Could you check a few things on this model? Use its own coordinates, in mm. A direction names the side the tool comes from. Coordinates: 2 decimals unless noted, no trailing zeros. Order: outer loops, then holes, each group sorted by start corner. A loop starts at its lowest first (then second) coordinate and runs counter-clockwise, first axis right, second up. Notation, with made-up numbers: (82.5, -23) - (99.5, -23) arc R29 cw to (99.5, 1) - close; hole circle Ø9 at (60.25, -35). An arc over 180 degrees is marked (long way). One line per item, written item: value. Start each with the question number.
from build123d import *

# Parameters (mm, degrees)
F1_DEPTH = 3
F2_D     = 3


# Not quite as in the source:
# - a feature names something its author has since deleted; it is built from what else it names


with BuildPart() as f1:
    # F0 (on Top) → F1 (new body)
    with BuildSketch(Plane.XY):
        Polygon((0, 31), (0, 0), (-35, 0), (-35, -15), (0, -15), (16, -15), (16, 31), align=None)
    extrude(amount=F1_DEPTH)

    # F2 (through all)
    with Locations(Plane(origin=(0, 0, 0), x_dir=(1, 0, 0), z_dir=(0, 0, -1))):
        with Locations((8, -8), (8, -22), (-10, 7.5), (-30, 7.5), (8, 6), (8, -26), (8, 10)):
            Hole(F2_D / 2)


solid = f1.part
Q1. I want a section at D-D on x = -21. Please give me the cut outline in (y, z), then the cut area to 3 significant figures.
Q2. I want a section at A-A on x = -30. Please give me the cut outline in (y, z).
Q3. If I drill on L1, parallel to Y at x = 8, z = 1.4; L2, parallel to Y at x = -30, z = 1.15; L3, parallel to X at y = -10, z = 0.7, over which ranges is the centre line in solid material (lowest first)?
Q4. I want a section at C-C on z = 2.1. Please give me the cut outline in (x, y).
Q5. Which directions (+Z, -Z, +X, -X, +Y, -Y) give clear straight access to the entire face, cutting with the end or side of a thin tool? Please do faces 5 (the flat face through (-17, 0, 1)), 6 (the cylindrical face through (8.195, 24.513, 1.521)).
Q6. We'd pull the mould along X, two halves only. Please class faces 1 (the flat face through (16, 8, 1)), 2 (the flat face through (0, 16, 1)), 3 (the flat face through (8, 31, 1)), 4 (the cylindrical face through (-28.5, -7.57, 1.52)): +X half, -X half, draft (parallel to the pull), parting line (faces both ways), or undercut.
Q7. I'm going to push flat-ended pins straight in: pin 1 (1.8 mm diameter, centred on x = 8, y = 8, fed in from -Z); pin 2 (0.9 mm diameter, centred on x = -11, z = 1, fed in from +Y). Where does each tip first touch, or does it pass through?
Q8. I want a section at B-B on y = 26. Please give me the cut outline in (x, z), then the cut area to 3 significant figures.
Values follow:
1. outline: (-15, 0) - (0, 0) - (0, 3) - (-15, 3) - close
1. area: 45.0 mm^2
2. outline: (-15, 0) - (-9, 0) - (-9, 3) - (-15, 3) - close; (-6, 0) - (0, 0) - (0, 3) - (-6, 3) - close
3. L1: y = -15 to -11.5, -8.5 to -7.5, -4.5 to 6.5, 9.5 to 20.5, 23.5 to 24.5, 27.5 to 31
3. L2: y = -15 to -9, -6 to 0
3. L3: x = -35 to 6.5, 9.5 to 16
4. outline: (-35, -15) - (16, -15) - (16, 31) - (0, 31) - (0, 0) - (-35, 0) - close; hole circle Ø3 at (-30, -7.5); hole circle Ø3 at (-10, -7.5); hole circle Ø3 at (8, -10); hole circle Ø3 at (8, -6); hole circle Ø3 at (8, 8); hole circle Ø3 at (8, 22); hole circle Ø3 at (8, 26)
5. face 5: +Z, -Z, -X, +Y
5. face 6: +Z, -Z
6. face 1: +X half
6. face 2: -X half
6. face 3: draft
6. face 4: undercut
7. pin 1: passes through
7. pin 2: stops at y = 0
8. outline: (0, 0) - (6.5, 0) - (6.5, 3) - (0, 3) - close; (9.5, 0) - (16, 0) - (16, 3) - (9.5, 3) - close
8. area: 39.0 mm^2
